from build123d import *

# Parameters (mm, degrees)
SKETCH1_W           = 101.6
SKETCH1_H           = 76.2
BOSS_EXTRUDE4_DEPTH = 12.7
BOSS_EXTRUDE5_DEPTH = 10.16
SKETCH5_R           = 3.175
CUT_EXTRUDE1_DEPTH  = 120.811560377
SKETCH6_R           = 6.35
CUT_EXTRUDE2_DEPTH  = 152.252681299
RIB1_REACH          = 132.755
SKETCH7_WALL_W      = 380.597220188
SKETCH7_WALL_H      = 12.7
FILLET2_R           = 2.54


with BuildPart() as part:
    # Sketch1 → Boss-Extrude4 (new body)
    with BuildSketch(Plane(origin=(0, 0, 0), x_dir=(1, 0, 0), z_dir=(0, 1, 0))):
        Rectangle(SKETCH1_W, SKETCH1_H)
    extrude(amount=BOSS_EXTRUDE4_DEPTH)

    # Sketch4 → Boss-Extrude5 (add)
    with BuildSketch(Plane.ZY.offset(50.8)):
        with BuildLine():
            Line((38.1, 0), (38.1, 76.2))
            ThreePointArc((38.1, 76.2), (0, 114.3), (-38.1, 76.2))
            Line((-38.1, 76.2), (-38.1, 0))
            Line((-38.1, 0), (38.1, 0))
        make_face()
    extrude(amount=-BOSS_EXTRUDE5_DEPTH)

    # Sketch5 → Cut-Extrude1 (cut, through all)
    with BuildSketch(Plane(origin=(0, 12.7, 0), x_dir=(1, 0, 0), z_dir=(0, 1, 0))):
        with Locations(Location((-25.4, 27.94, 0), (0, 0, 270))):
            Circle(SKETCH5_R)
        with Locations(Location((25.4, 27.94, 0), (0, 0, 270))):
            Circle(SKETCH5_R)
        with Locations(Location((25.4, 12.7, 0), (0, 0, 270))):
            Circle(SKETCH5_R)
        with Locations(Location((-25.4, 12.7, 0), (0, 0, 270))):
            Circle(SKETCH5_R)
        with BuildLine():
            Line((-25.4, -17.78), (0, -17.78))
            ThreePointArc((0, -17.78), (7.62, -25.4), (0, -33.02))
            Line((0, -33.02), (-25.4, -33.02))
            ThreePointArc((-25.4, -33.02), (-33.02, -25.4), (-25.4, -17.78))
        make_face()
    extrude(amount=-CUT_EXTRUDE1_DEPTH, mode=Mode.SUBTRACT)

    # Sketch6 → Cut-Extrude2 (cut, through all)
    with BuildSketch(Plane(origin=(-40.64, 0, 0), x_dir=(0, 0, -1), z_dir=(1, 0, 0))):
        with Locations((-25.4, 50.8)):
            Circle(SKETCH6_R)
        with Locations(Location((25.4, 50.8, 0), (0, 0, 180))):
            Circle(SKETCH6_R)
    extrude(amount=-CUT_EXTRUDE2_DEPTH, mode=Mode.SUBTRACT)

    # Sketch7 wall → Rib1 (add, up to next)
    with BuildSketch(Plane(origin=(-2.54, 57.15, 0), x_dir=(0.650791373456, -0.759256602365, 0), z_dir=(0.759256602365, 0.650791373456, 0)), mode=Mode.PRIVATE) as rib1_sk1:
        Rectangle(SKETCH7_WALL_W, SKETCH7_WALL_H)
    rib1_tool1 = extrude(rib1_sk1.sketch, amount=-RIB1_REACH, mode=Mode.PRIVATE) - part.part
    add(rib1_tool1.solids().sort_by_distance((-2.54, 57.15, 0))[0])

    # Fillet2
    fillet2_edges = [part.edges().sort_by_distance(p)[0] for p in [
        (-40.64, 12.7, 22.225),
        (-40.64, 12.7, -22.225),
        (-40.64, 57.15, -6.35),
        (-40.64, 57.15, 6.35),
    ]]
    fillet(fillet2_edges, radius=FILLET2_R)


solid = part.part
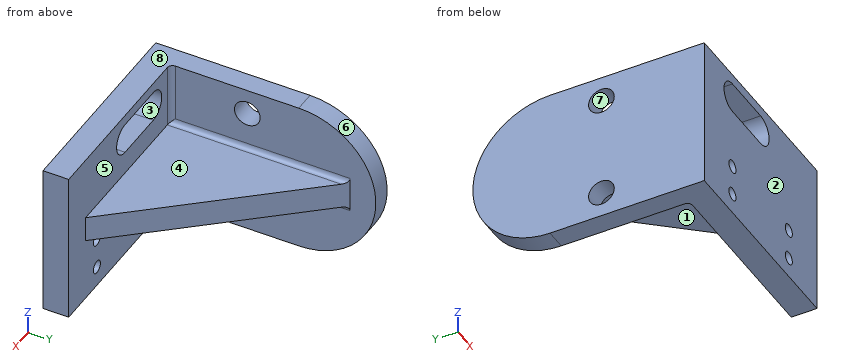
Design review of the part built by this model. Coordinates are the model's own, in mm. Face numbers are marked on the shaded views. A direction names the side the tool comes from. Round coordinates to 2 decimals unless told otherwise and drop trailing zeros. Write each loop counter-clockwise with the first axis right and the second up, starting at its lowest first coordinate (ties: lowest second). Pieces come first, ordered by that corner, then holes.
Item 1: For pin 1 Ø23 at (x, z) = (16.5, 2.5) entering from +Y; pin 2 Ø4 at (y, z) = (27.5, -12) entering from +X, all flat-tipped, find the tip position at first contact; note any pin that passes through.
Item 2: Consider section D-D on x = 13. Give the boundary of the cut face in (y, z), and give its area (3 significant figures).
Item 3: Consider section A-A on x = -12. Give the boundary of the cut face in (y, z), and give its area (3 significant figures).
Item 4: Wall thickness on L1, parallel to Z at x = -25, y = 10; L2, parallel to X at y = 8.5, z = -12.7 (3 decimals); L3, parallel to Z at x = -44, y = 50: over which ranges is each line inside the solid? List them lowest first.
Item 5: For the marked faces 1, 2, 3, 4 and 5, list the 3-axis set-ups (+Z, -Z, +X, -X, +Y, -Y) from which the entire face can be reached by the end or side of a thin tool; tool diameter is ignored.
Item 6: Consider section C-C on z = -12.7. Give the boundary of the cut face in (x, y) (3 decimals), and give its area (3 significant figures).
Item 7: Consider section B-B on z = 0. Give the boundary of the cut face in (x, y).
Item 8: Draft analysis for pull direction Y (two halves, no side actions). For the marked faces 6, 7 and 8, state which applies: released by +Y, released by -Y, zero draft, split by the parting line, or undercut.
Check values:
1. pin 1: stops at y = 48.35
1. pin 2: stops at x = -40.64
2. outline: (0, -38.1) - (12.7, -38.1) - (12.7, -6.35) - (39.02, -6.35) - (39.02, 6.35) - (12.7, 6.35) - (12.7, 38.1) - (0, 38.1) - close
2. area: 1,300 mm2
3. outline: (0, -38.1) - (12.7, -38.1) - (12.7, -6.35) - (68.19, -6.35) - (68.19, 6.35) - (12.7, 6.35) - (12.7, 17.78) - (0, 17.78) - close; (0, 33.02) - (12.7, 33.02) - (12.7, 38.1) - (0, 38.1) - close
3. area: 1,480 mm2
4. L1: z = -38.1 to -31.09, -24.79 to -15.85, -9.55 to 17.78, 33.02 to 38.1
4. L2: x = -50.8 to -28.575, -22.225 to 22.225, 28.575 to 50.8
4. L3: z = -38.1 to -31.7, -19.1 to 19.1, 31.7 to 38.1
5. face 1: -Z, +X, +Y
5. face 2: +Z, -Z, +X, -X, -Y
5. face 3: +Y, -Y
5. face 4: +Z, +X, +Y
5. face 5: +X, +Y
6. outline: (-50.8, 0) - (-28.575, 0) - (-28.575, 12.7) - (-38.1, 12.7) arc R2.54 cw to (-40.64, 15.24) - (-40.64, 112.121) - (-50.8, 112.121) - close; (-22.225, 0) - (22.225, 0) - (22.225, 12.7) - (-22.225, 12.7) - close; (28.575, 0) - (50.8, 0) - (50.8, 12.7) - (28.575, 12.7) - close
6. area: 2,140 mm2
7. outline: (-50.8, 0) - (50.8, 0) - (50.8, 12.7) - (35.56, 12.7) - (-40.64, 101.6) - (-40.64, 114.3) - (-50.8, 114.3) - close
8. face 6: released by +Y
8. face 7: undercut
8. face 8: zero draft
